Study the drawing (mm; zero at the part's minimum x, y, z) and answer. Coordinates: 2 decimals unless noted, no trailing zeros. Order: outer loops, then holes, each group sorted by start corner. A loop starts at its lowest first (then second) coordinate and runs counter-clockwise, first axis right, second up. Notation, with made-up numbers: M 32,-11.75 L 65,-11.75 A28 ccw 65,10.25 Z; hole C 81.25,-11.75 d3. An arc over 180 degrees is marked long. Use a Markdown table: item, result. Add a question column.
1) Each of these flat-tipped pins is pushed along its axis until it touches: pin 1 Ø8 at (y, z) = (30, 27) entering from -X; pin 2 Ø12 at (y, z) = (10.5, 27.5) entering from -X; pin 3 Ø10 at (x, z) = (40.5, 40.5) entering from +Y. Where does it stop, or does it pass through?
2) Find section B-B on z = 20. Write down the section's boundary in (x, y).
3) Find the intervals of material crossed by probe 1 along Y at (x, z) = (23, 15); probe 2 along X at (y, z) = (46.5, 3.5); probe 3 along X at (y, z) = (20, 14) (3 decimals), in increasing order. Write a range as [from, to].
4) Find section C-C on y = 36. Write down the section's boundary in (x, z), plus the area to 3 significant figures.
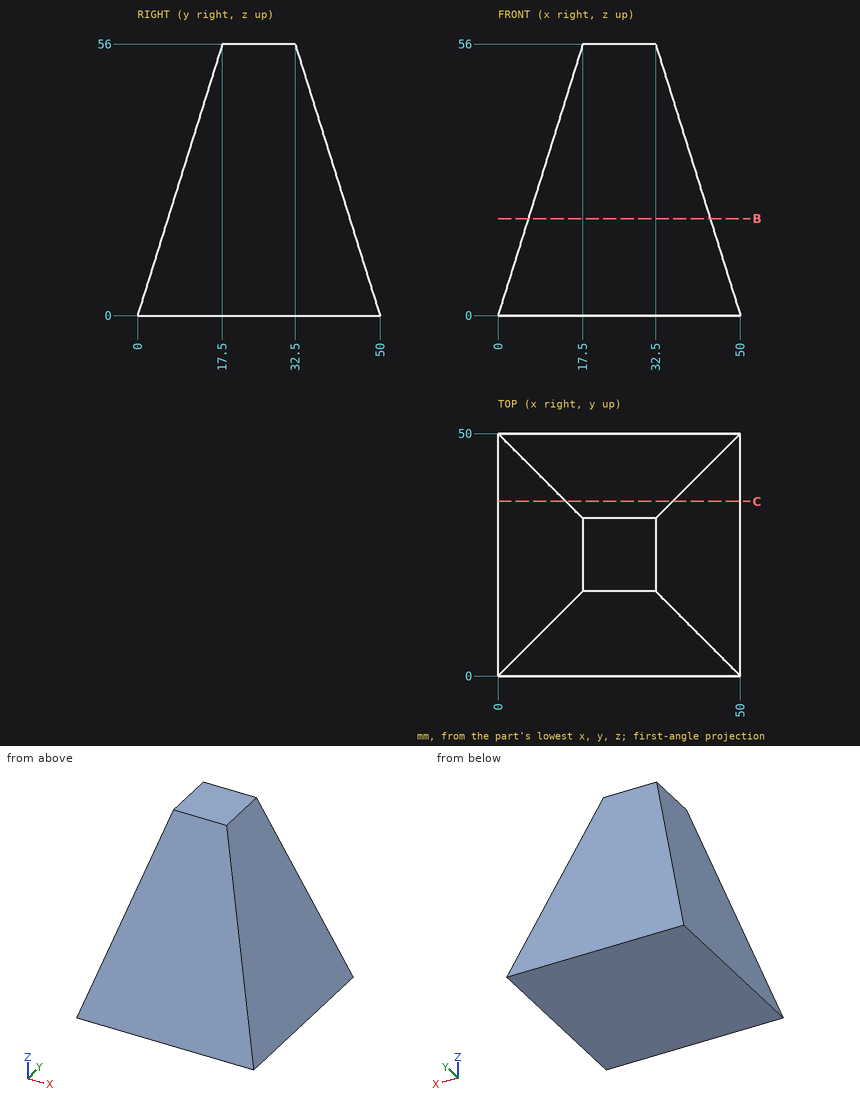
Check result:
| question | item | result |
|---|---|---|
| 1 | pin 1 | stops at x = 7.19 |
| 1 | pin 2 | stops at x = 6.72 |
| 1 | pin 3 | stops at y = 38.81 |
| 2 | outline | M 6.25,6.25 L 43.75,6.25 L 43.75,43.75 L 6.25,43.75 Z |
| 3 | probe 1 | y = [4.69, 45.31] |
| 3 | probe 2 | x = [1.09, 48.91] |
| 3 | probe 3 | x = [4.375, 45.625] |
| 4 | outline | M 0,0 L 50,0 L 36,44.8 L 14,44.8 Z |
| 4 | area | 1,610 mm2 |
